Input: part model. Units: mm. Frame: model coordinates. A direction names the side the tool comes from. Coordinates: 2 decimals unless noted, no trailing zeros. Loops run counter-clockwise (first coordinate to the right, second up) from the corner with the lowest first, then second, coordinate; pieces in that order, holes last.
```python
from build123d import *

# Parameters (mm, degrees)
F0_R     = 50
F1_DEPTH = 43
F2_R     = 144.3739928915
F2_R_2   = 50
F2_R_3   = 17
F3_DEPTH = 10
F4_R     = 61.7610309049
F5_DEPTH = 25
F6_R     = 10
F7_DEPTH = 12
F8_R     = 7.75
F9_DEPTH = 179


with BuildPart() as f1:
    # F0 (on Front) → F1 (new body)
    with BuildSketch(Plane.XZ):
        Circle(F0_R)
    extrude(amount=F1_DEPTH)

    # F2 (on face) → F3 (cut)
    with BuildSketch(Plane(origin=(0, 0, 0), x_dir=(-1, 0, 0), z_dir=(0, 1, 0))):
        Circle(F2_R)
        Circle(F2_R_2, mode=Mode.SUBTRACT)
        Circle(F2_R_2)
        Circle(F2_R_3, mode=Mode.SUBTRACT)
    extrude(amount=-F3_DEPTH, mode=Mode.SUBTRACT)

    # F4 (on face) → F5 (cut)
    with BuildSketch(Plane.XZ.offset(43)):
        Circle(F4_R)
    extrude(amount=-F5_DEPTH, mode=Mode.SUBTRACT)

    # F6 (on face) → F7 (cut)
    with BuildSketch(Plane.XZ.offset(18)):
        Circle(F6_R)
    extrude(amount=-F7_DEPTH, mode=Mode.SUBTRACT)

    # F8 (on Front) → F9 (cut)
    with BuildSketch(Plane.XZ):
        Circle(F8_R)
    extrude(amount=F9_DEPTH, mode=Mode.SUBTRACT)


solid = f1.part
```
Item 1: Reachability of faces 4 (the face through (-1.009, -2.958, 7.684)), 5 (the face through (1, -10, -22)), 6 (the face through (2.9, -6, -7.4)) from +Z, -Z, +X, -X, +Y, -Y: full face, straight path, thin tool, end or side. Return the list, or none.
Result:
face 4: +Y, -Y
face 5: +Y
face 6: -Y
Item 2: Section query D-D (z = 40). Output: boundary loops of the cut face in (x, y), then the cut area to 3 significant figures.
Result:
outline: (-30, -18) - (30, -18) - (30, -10) - (-30, -10) - close
area: 480 mm2
Item 3: Line query: L1, parallel to Z at x = 0, y = -3.35; L2, parallel to Z at x = 0, y = -11.75; L3, parallel to Y at x = 0.5, z = -23. Output: solid intervals per line, ascending.
Result:
L1: z = -17 to -7.75, 7.75 to 17
L2: z = -50 to -10, 10 to 50
L3: y = -18 to -10
Item 4: Contact query for flat-ended pins moving along their axis: P1, Ø6, axis at x = 0.5, z = 5, coming from the -Y side; P2, Ø12, axis at x = -11.5, z = -35.5, coming from the +Y side; P3, Ø1, axis at y = -16, z = 2, coming from the +X side; P4, Ø10, axis at x = 35.5, y = -4, coming from the +Z side. Output: stop coordinate, or through.
Result:
P1: stops at y = -6
P2: stops at y = -10
P3: stops at x = 49.98
P4: passes through
Item 5: Section query B-B (z = 0). Output: boundary loops of the cut face in (x, y), then the cut area to 3 significant figures.
Result:
outline: (-50, -18) - (-10, -18) - (-10, -6) - (-7.75, -6) - (-7.75, 0) - (-17, 0) - (-17, -10) - (-50, -10) - close; (7.75, -6) - (10, -6) - (10, -18) - (50, -18) - (50, -10) - (17, -10) - (17, 0) - (7.75, 0) - close
area: 807 mm2
Item 6: Section query A-A (x = 0). Output: boundary loops of the cut face in (y, z), then the cut area to 3 significant figures.
Result:
outline: (-18, -50) - (-10, -50) - (-10, -17) - (0, -17) - (0, -7.75) - (-6, -7.75) - (-6, -10) - (-18, -10) - close; (-18, 10) - (-6, 10) - (-6, 7.75) - (0, 7.75) - (0, 17) - (-10, 17) - (-10, 50) - (-18, 50) - close
area: 807 mm2
Item 7: Section query C-C (y = -8.75). Output: boundary loops of the cut face in (x, z).
Result:
outline: circle Ø34 at (0, 0); hole circle Ø20 at (0, 0)
Item 8: Mould query, pull axis X, two halves, no side actions, for faces 1 (the face through (7, 0, -4)), 2 (the face through (47.69, -13.94, 15.02)), 3 (the face through (-2.17, -12.08, -9.76)). Classes: +X half, -X half, draft (parallel to the pull), parting line (faces both ways), or undercut.
Result:
face 1: draft
face 2: parting line
face 3: undercut
